```python
from build123d import *

# Parameters (mm, degrees)
CYLINDER009_R         = 1.65
CYLINDER009_DEPTH     = 24
CYLINDER008_R         = 3.5
CYLINDER008_DEPTH     = 24
CHAMFER020026006_SIZE = 0.4


with BuildPart() as cylinder009:
    # Cylinder009 → Cylinder009 (new body)
    with BuildSketch(Plane(origin=(9, 39, 2), x_dir=(1, 0, 0), z_dir=(0, 0, 1))):
        Circle(CYLINDER009_R)
    extrude(amount=CYLINDER009_DEPTH)


with BuildPart() as chamfer020026006:
    # Cylinder008 → Cylinder008 (new body)
    with BuildSketch(Plane(origin=(9, 39, 2), x_dir=(1, 0, 0), z_dir=(0, 0, 1))):
        Circle(CYLINDER008_R)
    extrude(amount=CYLINDER008_DEPTH)

    # Cut002002002007004004001006014: cut Cylinder009
    add(cylinder009.part, mode=Mode.SUBTRACT)

    # Chamfer020026006
    chamfer020026006_edges = [chamfer020026006.edges().sort_by_distance(p)[0] for p in [
        (5.5, 39, 26),
        (5.5, 39, 2),
        (7.35, 39, 26),
        (7.35, 39, 2),
    ]]
    chamfer(chamfer020026006_edges, length=CHAMFER020026006_SIZE)


solid = chamfer020026006.part
```
Geometry check sheet. Reference: the model listing, model coordinates, mm. Give positions to 0.01 mm unless a question says otherwise; leave off trailing zeros. Write each loop counter-clockwise with the first axis right and the second up, starting at its lowest first coordinate (ties: lowest second). Pieces come first, ordered by that corner, then holes.
1) Section check B-B, the plane y = 39. Record the boundary of the cut face in (x, z), and give its area (3 significant figures).
2) Release check for a two-part mould opening along X. For faces 1 (the cylindrical face through (8.54, 42.47, 13.84)), 2 (the cylindrical face through (9.89, 40.39, 13.84)), 3 (the flat face through (10, 37, 26)) record: pulls with the +X half, pulls with the -X half, needs draft (parallel to the pull), parting line crosses it, or undercut.
3) Gauge pin test, flat ends, axial feed: pin 1 (1 mm diameter, centred on y = 38.5, z = 10.5, fed in from +X); pin 2 (3 mm diameter, centred on x = 9, y = 39, fed in from -Z); pin 3 (1 mm diameter, centred on x = 11, z = 5, fed in from -Y); pin 4 (1.5 mm diameter, centred on y = 38, z = 16.5, fed in from -X). Record the tip position at first contact, or that the pin passes through.
4) Section check A-A, the plane x = 9. Record the boundary of the cut face in (y, z), and give its area (3 significant figures).
5) Material ranges on L1, parallel to Y at x = 9, z = 8.75; L2, parallel to Y at x = 8, z = 16.5; L3, parallel to X at y = 40.25, z = 19.5, recorded low to high.
6) Section check C-C, the plane z = 20.5. Record the boundary of the cut face in (x, y).
Computed:
1. outline: (5.5, 2.4) - (5.9, 2) - (6.95, 2) - (7.35, 2.4) - (7.35, 25.6) - (6.95, 26) - (5.9, 26) - (5.5, 25.6) - close; (10.65, 2.4) - (11.05, 2) - (12.1, 2) - (12.5, 2.4) - (12.5, 25.6) - (12.1, 26) - (11.05, 26) - (10.65, 25.6) - close
1. area: 88.2 mm2
2. face 1: parting line crosses it
2. face 2: undercut
2. face 3: needs draft
3. pin 1: stops at x = 12.5
3. pin 2: passes through
3. pin 3: stops at y = 35.84
3. pin 4: stops at x = 5.51
4. outline: (35.5, 2.4) - (35.9, 2) - (36.95, 2) - (37.35, 2.4) - (37.35, 25.6) - (36.95, 26) - (35.9, 26) - (35.5, 25.6) - close; (40.65, 2.4) - (41.05, 2) - (42.1, 2) - (42.5, 2.4) - (42.5, 25.6) - (42.1, 26) - (41.05, 26) - (40.65, 25.6) - close
4. area: 88.2 mm2
5. L1: y = 35.5 to 37.35, 40.65 to 42.5
5. L2: y = 35.65 to 37.69, 40.31 to 42.35
5. L3: x = 5.73 to 7.92, 10.08 to 12.27
6. outline: circle Ø7 at (9, 39); hole circle Ø3.3 at (9, 39)
